Autodesk Inventor part; units mm, degrees
ref_plane "YZ Plane" through (0, 0, 0) normal (1, 0, 0) x (0, 1, 0)
ref_plane "XZ Plane" through (0, 0, 0) normal (0, 1, 0) x (-1, 0, 0)
ref_plane "XY Plane" through (0, 0, 0) normal (0, 0, 1) x (1, 0, 0)
sketch "Sketch1" plane through (0, 0, 0) normal (0, 1, 0) x (-1, 0, 0)
  line L0 (11.5, 24) -> (-11.5, 24)
  line L1 (-11.5, 24) -> (-11.5, -24)
  line L2 (-11.5, -24) -> (11.5, -24)
  line L3 (11.5, -24) -> (11.5, 24)
  line L4 (11.5, 24) -> (-11.5, -24) construction
  line L5 (-11.5, 24) -> (11.5, -24) construction
  line L6 (-8.5, 21) -> (8.5, 21)
  line L7 (8.5, 21) -> (8.5, -21)
  line L8 (8.5, -21) -> (-8.5, -21)
  line L9 (-8.5, -21) -> (-8.5, 21)
  line L10 (-8.5, 21) -> (8.5, -21) construction
  line L11 (8.5, 21) -> (-8.5, -21) construction
  line L12 (0, 0) -> (-8.5, 0) construction
  circle A0 centre (0, -12) radius 1.5
  circle A1 centre (0, 12) radius 1.5
  line L13 (17.5, 30) -> (-17.5, 30)
  line L14 (-17.5, 30) -> (-17.5, -30)
  line L15 (-17.5, -30) -> (17.5, -30)
  line L16 (17.5, -30) -> (17.5, 30)
  line L17 (17.5, 30) -> (-17.5, -30) construction
  line L18 (-17.5, 30) -> (17.5, -30) construction
  dimension "d0" = 23
  dimension "d1" = 48
  dimension "d3" = 3
  dimension "d4" = 3
  dimension "d5" = 3
  dimension "d6" = 12
  dimension "d9" = 6
  dimension "d10" = 6
extrude "Extrusion1" add sketch "Sketch1" along normal blind 3 contours L6 L7 L8 L9
fillet "Fillet1" radius 1.5 4 edges at (8.5, 1.5, 21) (8.5, 1.5, -21) (-8.5, 1.5, 21) (-8.5, 1.5, -21)
properties part number "Middle internal"
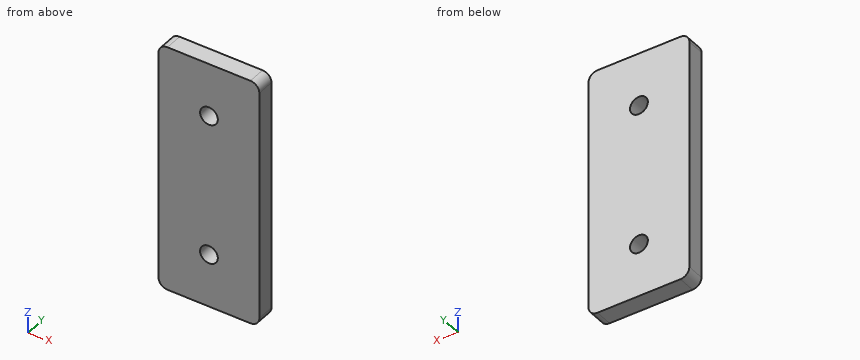
The model under review builds one solid part; all positions refer to its coordinate system, in mm. Round coordinates to 2 decimals unless told otherwise and drop trailing zeros. Loops run counter-clockwise (first coordinate to the right, second up) from the corner with the lowest first, then second, coordinate; pieces in that order, holes last.
Item 1: Take a section at D-D (z = 11.5). Write out the cut boundary in (x, y), then the cut area to 3 significant figures.
Determined:
outline: (-8.5, 0) - (-1.41, 0) - (-1.41, 3) - (-8.5, 3) - close; (1.41, 0) - (8.5, 0) - (8.5, 3) - (1.41, 3) - close
area: 42.5 mm2
Item 2: For line 1 (Z direction, x = 0, y = 1.7); line 2 (Z direction, x = -0.5, y = 0.85); line 3 (X direction, y = 1.4, z = 13), list the stretches that pass through material, from the lowest coordinate up.
Determined:
line 1: z = -21 to -13.5, -10.5 to 10.5, 13.5 to 21
line 2: z = -21 to -13.41, -10.59 to 10.59, 13.41 to 21
line 3: x = -8.5 to -1.12, 1.12 to 8.5
Item 3: Clearance check with a flat-ended pin moving along its axis: pin 1 Ø1.8 at (x, z) = (0, 12) entering from +Y. State where the tip first meets the part, or that it passes through.
Determined:
pin 1: passes through
Item 4: Take a section at C-C (y = 2.5). Write out the cut boundary in (x, z), then the cut area to 3 significant figures.
Determined:
outline: (-8.5, -19.5) arc R1.5 ccw to (-7, -21) - (7, -21) arc R1.5 ccw to (8.5, -19.5) - (8.5, 19.5) arc R1.5 ccw to (7, 21) - (-7, 21) arc R1.5 ccw to (-8.5, 19.5) - close; hole circle Ø3 at (0, -12); hole circle Ø3 at (0, 12)
area: 698 mm2
Item 5: Take a section at A-A (x = 0). Write out the cut boundary in (y, z).
Determined:
outline: (0, -21) - (3, -21) - (3, -13.5) - (0, -13.5) - close; (0, -10.5) - (3, -10.5) - (3, 10.5) - (0, 10.5) - close; (0, 13.5) - (3, 13.5) - (3, 21) - (0, 21) - close
Item 6: Take a section at B-B (z = -12). Write out the cut boundary in (x, y), then the cut area to 3 significant figures.
Determined:
outline: (-8.5, 0) - (-1.5, 0) - (-1.5, 3) - (-8.5, 3) - close; (1.5, 0) - (8.5, 0) - (8.5, 3) - (1.5, 3) - close
area: 42.0 mm2
